Autodesk Inventor part; units mm, degrees
ref_plane "YZ Plane" through (0, 0, 0) normal (1, 0, 0) x (0, 1, 0)
ref_plane "XZ Plane" through (0, 0, 0) normal (0, 1, 0) x (-1, 0, 0)
ref_plane "XY Plane" through (0, 0, 0) normal (0, 0, 1) x (1, 0, 0)
sketch "Esquisse1" plane through (0, 0, 0) normal (0, 0, 1) x (1, 0, 0)
  line L0 (0, 0) -> (125, 0)
  line L1 (125, 0) -> (125, 150)
  line L2 (125, 150) -> (0, 150)
  line L3 (0, 150) -> (0, 0)
  dimension "d0" = 125
  dimension "d1" = 150
extrude "Extrusion1" add sketch "Esquisse1" along normal blind 3
sketch "Esquisse2" plane through (0, 0, 3) normal (0, 0, 1) x (1, 0, 0)
  circle A0 centre (65, 70) radius 35
  line L0 (125, 0) -> (125, 150)
  line L1 (125, 150) -> (0, 150)
  point P0 (0, 0)
  dimension "d4" = 70
  dimension "d5" = 60
  dimension "d6" = 80
extrude "Extrusion2" cut sketch "Esquisse2" against normal blind 3
properties part number "cale-moteur"
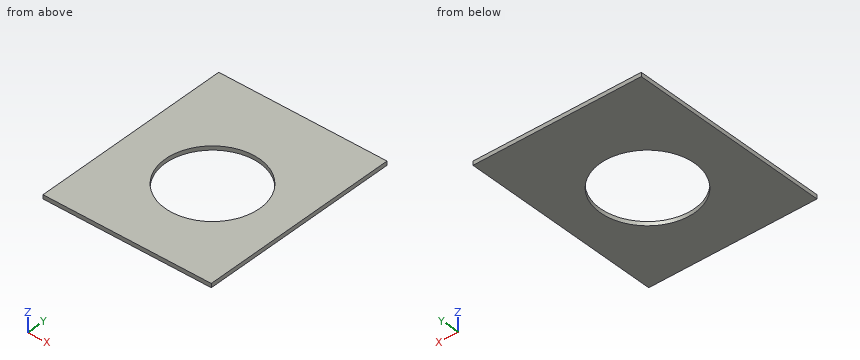
Read the model definition and answer for the solid it produces. Units are mm, in the model's axes. Coordinates: 2 decimals unless noted, no trailing zeros. Loops run counter-clockwise (first coordinate to the right, second up) from the corner with the lowest first, then second, coordinate; pieces in that order, holes last.
Q1. The part is cut by section B-B on x = 65. Write down the section's boundary in (y, z), and give its area (3 significant figures).
Q2. The part is cut by section A-A on y = 70. Write down the section's boundary in (x, z), and give its area (3 significant figures).
Q3. The part is cut by section C-C on z = 1.95. Write down the section's boundary in (x, y).
Q4. Consider probe 1 along X at (y, z) = (71, 1.2); probe 2 along Y at (x, z) = (65, 2.4); probe 3 along X at (y, z) = (38.5, 1.25). Determine where each line is inside the solid, lowest interval first.
Results below:
1. outline: (0, 0) - (35, 0) - (35, 3) - (0, 3) - close; (105, 0) - (150, 0) - (150, 3) - (105, 3) - close
1. area: 240 mm2
2. outline: (0, 0) - (30, 0) - (30, 3) - (0, 3) - close; (100, 0) - (125, 0) - (125, 3) - (100, 3) - close
2. area: 165 mm2
3. outline: (0, 0) - (125, 0) - (125, 150) - (0, 150) - close; hole circle Ø70 at (65, 70)
4. probe 1: x = 0 to 30.01, 99.99 to 125
4. probe 2: y = 0 to 35, 105 to 150
4. probe 3: x = 0 to 49.74, 80.26 to 125
